from build123d import *

# Parameters (mm, degrees)
F2_R      = 76.2
F5_DEPTH  = 609.6
F4_R      = 76.2
F6_DEPTH  = 304.8
F7_T      = -25.4
F7_2_T    = -25.4
F9_R      = 95.25
F9_R_2    = 76.2
F10_DEPTH = 25.4
F12_R     = 95.25
F12_R_2   = 76.2
F13_DEPTH = 25.4
F14_R     = 95.25
F14_R_2   = 76.2
F15_DEPTH = 25.4


with BuildPart() as f5:
    # F2 (on plane+point) → F5 (new body)
    with BuildSketch(Plane.XZ.offset(294.1361665726)):
        Circle(F2_R)
    extrude(amount=-F5_DEPTH)

    # F7
    f7_openings = [f5.faces().sort_by_distance(p)[0] for p in [
        (0, 315.463833, 0),
        (0, -294.136167, 0),
    ]]
    offset(amount=F7_T, openings=f7_openings)

    # F9 (on line) → F10 (join)
    with BuildSketch(Plane(origin=(0, -294.1361665726, 0), x_dir=(-1, 0, 0), z_dir=(0, 1, 0))):
        Circle(F9_R)
        Circle(F9_R_2, mode=Mode.SUBTRACT)
    extrude(amount=F10_DEPTH)

    # F12 (on line) → F13 (join)
    with BuildSketch(Plane(origin=(0, 315.4638334274, 0), x_dir=(-1, 0, 0), z_dir=(0, 1, 0))):
        Circle(F12_R)
        Circle(F12_R_2, mode=Mode.SUBTRACT)
    extrude(amount=-F13_DEPTH)



with BuildPart() as f6:
    # F4 (on plane+point) → F6 (new body)
    with BuildSketch(Plane.XY.offset(304.8)):
        Circle(F4_R)
    extrude(amount=-F6_DEPTH)

    # F7#2
    f7_2_openings = [f6.faces().sort_by_distance(p)[0] for p in [
        (0, 0, 304.8),
    ]]
    offset(amount=F7_2_T, openings=f7_2_openings)


with BuildPart() as f5_1:
    add(f5.part)

    add(f6.part)  # F15 merges F6
    # F14 (on plane+point) → F15 (join)
    with BuildSketch(Plane.XY.offset(304.8)):
        Circle(F14_R)
        Circle(F14_R_2, mode=Mode.SUBTRACT)
    extrude(amount=-F15_DEPTH)


solid = f5_1.part
Input: part model. Units: mm. Frame: model coordinates. A direction names the side the tool comes from. Give positions to 0.01 mm unless a question says otherwise; leave off trailing zeros. Order: outer loops, then holes, each group sorted by start corner. A loop starts at its lowest first (then second) coordinate and runs counter-clockwise, first axis right, second up.
Q1. Section A-A on y = 0. Output: boundary loops of the cut face in (x, z), and give its area (3 significant figures).
Checked values:
outline: (-95.25, 279.4) - (-76.2, 279.4) - (-76.2, 0) arc R76.2 ccw to (76.2, 0) - (76.2, 279.4) - (95.25, 279.4) - (95.25, 304.8) - (50.8, 304.8) - (50.8, 56.8) arc R76.2 ccw to (-50.8, 56.8) - (-50.8, 304.8) - (-95.25, 304.8) - close; hole (-50.8, 0) arc R50.8 ccw to (50.8, 0) - close; hole (-43.99, 25.4) - (43.99, 25.4) arc R50.8 ccw to start
area: 27,100 mm2
Q2. Ray query, probe 1 along Y at (x, z) = (0, 230); probe 2 along Z at (x, y) = (0, 44); probe 3 along Y at (x, z) = (-48.5, -66.5). Return the intervals inside material, ascending.
Checked values:
probe 1: y = -76.2 to -50.8, 50.8 to 76.2
probe 2: z = -76.2 to -50.8, 0 to 25.4, 50.8 to 76.2
probe 3: y = -294.14 to -268.74, 290.06 to 315.46
Q3. Draft query along X for faces 6 (the cylindrical face through (0.778, 76.196, 20.112)), 7 (the cylindrical face through (-60.47, -46.367, 172.7)), 8 (the flat face through (43, -268.736, 64)). Return one class per face: +X half, -X half, draft (parallel to the pull), parting line (faces both ways), or undercut.
Checked values:
face 6: undercut
face 7: parting line
face 8: draft
Q4. Section C-C on z = 86.5. Output: boundary loops of the cut face in (x, y), and give its area (3 significant figures).
Checked values:
outline: circle Ø152.4 at (0, 0); (-39.88, -294.14) - (39.88, -294.14) - (39.88, -268.74) - (-39.88, -268.74) - close; (-39.88, 290.06) - (39.88, 290.06) - (39.88, 315.46) - (-39.88, 315.46) - close; hole circle Ø101.6 at (0, 0)
area: 14,200 mm2
Q5. Set-up query: faces 1 (the flat face through (-1, 1, 0)), 2 (the cylindrical face through (75.587, 302.942, -57.958)), 3 (the cylindrical face through (-75.587, -57.958, 292.278)), 4 (the cylindrical face through (-11.012, 6.397, -49.592)), 5 (the cylindrical face through (75.587, -281.614, -57.958)). Return all of +Z, -Z, +X, -X, +Y, -Y with unobstructed straight access to the full face (end or side cutting, diameter ignored); none if empty.
Checked values:
face 1: +Y, -Y
face 2: +Y
face 3: +Z
face 4: none
face 5: -Y
Q6. Section D-D on z = 268. Output: boundary loops of the cut face in (x, y), and give its area (3 significant figures).
Checked values:
outline: circle Ø152.4 at (0, 0); hole circle Ø101.6 at (0, 0)
area: 10,100 mm2
Q7. Section B-B on x = 0. State how many separate pieces and enclosed holes the cut face has, and give its area (3 significant figures).
Checked values:
separate pieces: 2
enclosed holes: 1
area: 50,600 mm2
Q8. Contact query for flat-ended pins moving along their axis: pin 1 Ø3 at (x, y) = (-25, 206.5) entering from -Z; pin 2 Ø3 at (x, y) = (-39, 24.5) entering from -Z; pin 3 Ø12 at (x, y) = (18, -5) entering from -Z. Output: stop coordinate, or through.
Checked values:
pin 1: stops at z = -72.49
pin 2: stops at z = -66.33
pin 3: stops at z = -75.25
